Check sheet for the modelled part. Datum: model origin and axes. Units: mm. A direction names the side the tool comes from. Round coordinates to 2 decimals unless told otherwise and drop trailing zeros. Write each loop counter-clockwise with the first axis right and the second up, starting at its lowest first coordinate (ties: lowest second). Pieces come first, ordered by that corner, then holes. Notation, with made-up numbers: M 73,-24.75 L 98,-24.75 A10 ccw 98,-12.75 Z; hole C -18,59.5 d5. An arc over 180 degrees is marked long. Answer in a Markdown table with one row per item.
```python
from build123d import *

# Parameters (mm, degrees)
BOSS_EXTRUDE1_DEPTH     = 19.7
CUT_EXTRUDE1_DEPTH      = 128.410635349
CUT_EXTRUDE1_DEPTH_BACK = 128.410635349
SKETCH2_W               = 4
SKETCH2_H               = 6


with BuildPart() as part:
    # Sketch1 → Boss-Extrude1 (new body)
    with BuildSketch(Plane.XY):
        with BuildLine():
            Line((-115.3, 0), (-120, 0))
            ThreePointArc((-120, 0), (-122.355151556, 0.077929384), (-124.7, 0.311376618))
            Line((-124.7, 0.311376618), (-124.7, 1.924264069))
            Line((-124.7, 1.924264069), (-125.7, 2.924264069))
            Line((-125.7, 2.924264069), (-125.7, 3.675735931))
            Line((-125.7, 3.675735931), (-124.875735931, 4.5))
            Line((-124.875735931, 4.5), (-122, 4.5))
            Line((-122, 4.5), (-122, 6.7))
            Line((-122, 6.7), (-118, 6.7))
            Line((-118, 6.7), (-118, 4.5))
            Line((-118, 4.5), (-115.124264069, 4.5))
            Line((-115.124264069, 4.5), (-114.3, 3.675735931))
            Line((-114.3, 3.675735931), (-114.3, 2.924264069))
            Line((-114.3, 2.924264069), (-115.3, 1.924264069))
            Line((-115.3, 1.924264069), (-115.3, 0))
        make_face()
    extrude(amount=-BOSS_EXTRUDE1_DEPTH)

    # Sketch2 → Cut-Extrude1 (cut, two sides: drawn at the far end of the back side and taken through both)
    with BuildSketch(Plane(origin=(0, 6.7, 0), x_dir=(1, 0, 0), z_dir=(0, 1, 0)).offset(-CUT_EXTRUDE1_DEPTH_BACK)):
        with Locations((-120, 16.7)):
            Rectangle(SKETCH2_W, SKETCH2_H)
    extrude(amount=CUT_EXTRUDE1_DEPTH + CUT_EXTRUDE1_DEPTH_BACK, mode=Mode.SUBTRACT)


solid = part.part
```
1. Section check A-A, the plane z = -17.5. Record the cut outline in (x, y).
Found:
| item | result |
|---|---|
| outline | M -125.7,2.92 L -124.7,1.92 L -124.7,0.31 A35.63 ccw -122,0.06 L -122,4.5 L -124.88,4.5 L -125.7,3.68 Z; M -118,0 L -115.3,0 L -115.3,1.92 L -114.3,2.92 L -114.3,3.68 L -115.12,4.5 L -118,4.5 Z |
2. Section check B-B, the plane y = 1.5. Record the cut outline in (x, z), and give its area (3 significant figures).
Found:
| item | result |
|---|---|
| outline | M -124.7,-19.7 L -122,-19.7 L -122,-13.7 L -118,-13.7 L -118,-19.7 L -115.3,-19.7 L -115.3,0 L -124.7,0 Z |
| area | 161 mm2 |
3. Section check C-C, the plane z = -12.75. Record the cut outline in (x, y).
Found:
| item | result |
|---|---|
| outline | M -125.7,2.92 L -124.7,1.92 L -124.7,0.31 A35.63 ccw -120,0 L -115.3,0 L -115.3,1.92 L -114.3,2.92 L -114.3,3.68 L -115.12,4.5 L -118,4.5 L -118,6.7 L -122,6.7 L -122,4.5 L -124.88,4.5 L -125.7,3.68 Z |
4. Section check D-D, the plane x = -119. Record the cut outline in (y, z).
Found:
| item | result |
|---|---|
| outline | M 0,-13.7 L 6.7,-13.7 L 6.7,0 L 0,0 Z |
5. Access from +Z, -Z, +X, -X, +Y, -Y to the whole of each face (thin tool, end or side, straight path). Record for faces 5 (the face through (-115.3, 1, -10)), 6 (the face through (-118, 2, -17)), 7 (the face through (-123, 4.5, -10)), 8 (the face through (-120, 6.7, -7)).
Found:
| item | result |
|---|---|
| face 5 | +Z, -Z, +X, -Y |
| face 6 | -Z, +Y, -Y |
| face 7 | +Z, -Z, -X, +Y |
| face 8 | +Z, -Z, +X, -X, +Y |
6. Draft check along X on faces 1 (the face through (-120, 3, -13.7)), 2 (the face through (-117, 4.5, -10)), 3 (the face through (-124.7, 1, -10)), 4 (the face through (-118, 6, -7)). Enter one of: +X half, -X half, draft (parallel to the pull), parting line (faces both ways), or undercut.
Found:
| item | result |
|---|---|
| face 1 | undercut |
| face 2 | draft |
| face 3 | -X half |
| face 4 | +X half |
7. Go/stop test with flat-tipped pins: pin 1 (1 mm diameter, centred on y = 1, z = -5, fed in from +X); pin 2 (0.7 mm diameter, centred on y = 5.5, z = -4.5, fed in from +X); pin 3 (1.4 mm diameter, centred on x = -123, z = -11, fed in from +Y). Record where each tip stops, or that it passes through.
Found:
| item | result |
|---|---|
| pin 1 | stops at x = -115.3 |
| pin 2 | stops at x = -118 |
| pin 3 | stops at y = 4.5 |
8. Scan lines: L1, parallel to X at y = 1, z = -18.25; L2, parallel to X at y = 3.25, z = -18.25; L3, parallel to Z at x = -120, y = 3.75. Record each from-to range of solid material in increasing order.
Found:
| item | result |
|---|---|
| L1 | x = -124.7 to -122, -118 to -115.3 |
| L2 | x = -125.7 to -122, -118 to -114.3 |
| L3 | z = -13.7 to 0 |
